Work out the finished part from the listing and answer in its coordinate system (mm). A direction names the side the tool comes from. Coordinates: 2 decimals unless noted, no trailing zeros. Order: outer loops, then holes, each group sorted by start corner. A loop starts at its lowest first (then second) coordinate and runs counter-clockwise, first axis right, second up. Notation, with made-up numbers: (-27, -40) -> (-22, -40) arc R10 cw to (-22, -31) -> close; hole circle Ø9 at (60, -10.5). An arc over 180 degrees is marked (long way). Write item = value, one per line. Start each with the question number.
Q1. Straight lines are drawn through the part: L1, parallel to Z at x = 0, y = -2; L2, parallel to Z at x = 3, y = -2.75; L3, parallel to Y at x = 4.5, z = -16.5. For each, find the intervals that lie inside material, in ascending order. Write a range as from..to.
Q2. The part is cut by section C-C, the plane y = 3. Determine the outline of the cut face in (x, z).
Q3. The part is cut by section D-D, the plane z = 15. Determine the outline of the cut face in (x, y).
Q4. Which of the six approach directions +Z, -Z, +X, -X, +Y, -Y give full straight-line access (tool end or side, diameter ignored) to faces 4 (the flat face through (-5, -11, 9)), 5 (the cylindrical face through (-2.17, -7.06, -9.76))?
Q5. For a pull along Z with two mould halves and no side action, classify faces 1 (the cylindrical face through (-3, 4, 0)), 2 (the flat face through (0, -3, 0)), 3 (the flat face through (4, 0, 0)) as +Z half, -Z half, draft (parallel to the pull), parting line (faces both ways), or undercut.
Q6. Flat-ended cylindrical pins translate along their axes: pin 1 (8 mm diameter, centred on x = 4, z = -12.5, fed in from +Y); pin 2 (2.5 mm diameter, centred on x = -4.31, z = -4.07, fed in from -Y); pin 3 (10 mm diameter, centred on x = 12.5, y = -4, fed in from -Z); pin 4 (4 mm diameter, centred on x = -4.48, z = 4.32, fed in from -Y). Find the tip coordinate at first contact, or state that the pin passes through.
Q7. The part is cut by section A-A, the plane x = 0. Determine the outline of the cut face in (y, z).
Q8. The part is cut by section B-B, the plane y = -8.25. Determine the outline of the cut face in (x, z), plus the area to 3 significant figures.
```python
from build123d import *

# Parameters (mm, degrees)
F0_R     = 3
F1_DEPTH = 9
F2_R     = 3
F3_DEPTH = 9.5
F2_R_2   = 20
F4_DEPTH = 11
F5_R     = 10
F6_DEPTH = 8
F7_R     = 1.5
F8_DEPTH = 8


with BuildPart() as f1:
    # F0 (on Front) → F1 (new body)
    with BuildSketch(Plane.XZ):
        Circle(F0_R)
    extrude(amount=-F1_DEPTH)

    # F2 (on face) → F3 (join)
    with BuildSketch(Plane.XZ):
        Circle(F2_R)
    extrude(amount=F3_DEPTH)

    # F2 (on face) → F4 (join)
    with BuildSketch(Plane.XZ):
        Circle(F2_R_2)
    extrude(amount=F4_DEPTH)

    # F5 (on face) → F6 (cut)
    with BuildSketch(Plane.XZ.offset(11)):
        Circle(F5_R)
    extrude(amount=-F6_DEPTH, mode=Mode.SUBTRACT)

    # F7 (on face) → F8 (cut)
    with BuildSketch(Plane.XZ.offset(3)):
        with Locations((6.463317, -0.03593)):
            Circle(F7_R)
        with Locations((4.35309, 4.115115)):
            Circle(F7_R)
        with Locations((0, 6.331937)):
            Circle(F7_R)
        with Locations((-4.484795, 4.320276)):
            Circle(F7_R)
        with Locations((-6.611656, -0.013489)):
            Circle(F7_R)
        with Locations((-4.305509, -4.068238)):
            Circle(F7_R)
        with Locations((0.001843, -6.426248)):
            Circle(F7_R)
        with Locations((4.135434, -4.499229)):
            Circle(F7_R)
    extrude(amount=-F8_DEPTH, mode=Mode.SUBTRACT)


solid = f1.part
```
Model answer:
q1.L1 = -20..-7.93, -4.93..4.83, 7.83..20
q1.L2 = -19.77..-5.48, -3.52..3.47, 4.76..19.77
q1.L3 = -11..0
q2.outline = circle Ø6 at (0, 0)
q3.outline = (-13.23, -11) -> (13.23, -11) -> (13.23, 0) -> (-13.23, 0) -> close
q4.face_4 = +Z, -Z, +X, -X, -Y
q4.face_5 = -Y
q5.face_1 = parting line
q5.face_2 = undercut
q5.face_3 = draft
q6.pin_1 = 0
q6.pin_2 = through
q6.pin_3 = -18.54
q6.pin_4 = -3
q7.outline = (-11, -20) -> (0, -20) -> (0, -7.93) -> (-3, -7.93) -> (-3, -10) -> (-11, -10) -> close; (-11, 10) -> (-3, 10) -> (-3, 7.83) -> (0, 7.83) -> (0, 20) -> (-11, 20) -> close; (-3, -4.93) -> (0, -4.93) -> (0, -3) -> (9, -3) -> (9, 3) -> (0, 3) -> (0, 4.83) -> (-3, 4.83) -> close
q8.outline = circle Ø40 at (0, 0); hole circle Ø20 at (0, 0)
q8.area = 942 mm2
